Autodesk Inventor part; units mm, degrees
ref_plane "Work Plane1" through (0, 7.749, 0) normal (0, 1, 0) x (-1, 0, 0)
ref_plane "Work Plane2" through (0, 16.1, 0) normal (0, 1, 0) x (-1, 0, 0)
ref_plane "Work Plane3" through (0, 113.3, 0) normal (0, 1, 0) x (-1, 0, 0)
sketch "Sketch1" plane through (0, 0, 0) normal (0, 1, 0) x (-1, 0, 0)
  circle A0 centre (0, 0) radius 28.5
  circle A1 centre (0, 0) radius 31.877
  dimension "d0" = 57
  dimension "d1" = 63.754
extrude "Extrusion1" add sketch "Sketch1" along normal blind 114.2
ref_plane "Work Plane1" through (0, 7.749, 0) normal (0, 1, 0) x (-1, 0, 0)
sketch "Sketch3" plane through (0, 7.749, 0) normal (0, 1, 0) x (-1, 0, 0)
  circle A0 centre (0, 0) radius 31.877
  circle A1 centre (0, 0) radius 30.988
  dimension "d6" = 61.976
extrude "Extrusion2" cut sketch "Sketch3" along normal blind 200
ref_plane "Work Plane2" through (0, 16.1, 0) normal (0, 1, 0) x (-1, 0, 0)
sketch "Sketch4" plane through (0, 16.1, 0) normal (0, 1, 0) x (-1, 0, 0)
  circle A0 centre (0, 0) radius 29.5
  circle A1 centre (0, 0) radius 27.8909
  circle A2 centre (0, 0) radius 33.2417
  dimension "d10" = 59
extrude "Extrusion3" cut sketch "Sketch4" along normal blind 200 contours A2
ref_plane "Work Plane3" through (0, 113.3, 0) normal (0, 1, 0) x (-1, 0, 0)
properties part number "Vacuum Cylinder"
The listing builds one solid part. Answer for the finished solid, in the listing's coordinates (mm). A direction names the side the tool comes from. Round coordinates to 2 decimals unless told otherwise and drop trailing zeros. Order: outer loops, then holes, each group sorted by start corner. A loop starts at its lowest first (then second) coordinate and runs counter-clockwise, first axis right, second up. Notation, with made-up numbers: (29.5, 77) -> (54.5, 77) arc R22 cw to (54.5, 102) -> close; hole circle Ø6 at (35, -11.5). An arc over 180 degrees is marked (long way). Put each result on its own line as item: value.
Q1. Section B-B, the plane x = 0 is taken. Write down the section's boundary in (y, z).
Results list:
outline: (0, -31.88) -> (7.75, -31.88) -> (7.75, -30.99) -> (16.1, -30.99) -> (16.1, -29.5) -> (114.2, -29.5) -> (114.2, -28.5) -> (0, -28.5) -> close; (0, 28.5) -> (114.2, 28.5) -> (114.2, 29.5) -> (16.1, 29.5) -> (16.1, 30.99) -> (7.75, 30.99) -> (7.75, 31.88) -> (0, 31.88) -> close
Q2. Section A-A, the plane z = 0 is taken. Write down the section's boundary in (x, y).
Results list:
outline: (-31.88, 0) -> (-28.5, 0) -> (-28.5, 114.2) -> (-29.5, 114.2) -> (-29.5, 16.1) -> (-30.99, 16.1) -> (-30.99, 7.75) -> (-31.88, 7.75) -> close; (28.5, 0) -> (31.88, 0) -> (31.88, 7.75) -> (30.99, 7.75) -> (30.99, 16.1) -> (29.5, 16.1) -> (29.5, 114.2) -> (28.5, 114.2) -> close
Q3. Each of these flat-tipped pins is pushed along its axis until it touches: P1, Ø4, axis at y = 31.5, z = 18, coming from the +X side; P2, Ø4, axis at x = 18, y = 76, coming from the +Z side; P3, Ø1.5, axis at x = -3.5, y = 100.5, coming from the +Z side; P4, Ø10, axis at x = -3, z = 20, coming from the -Y side. Where does it stop, or does it pass through?
Results list:
P1: x = 24.78
P2: z = 24.78
P3: z = 29.37
P4: through
Q4. Section C-C, the plane y = 49 is taken. Write down the section's boundary in (x, z), and give its area (3 significant figures).
Results list:
outline: circle Ø59 at (0, 0); hole circle Ø57 at (0, 0)
area: 182 mm^2
Q5. Consider line 1 along Z through (x, y) = (0, 72.5); line 2 along X through (y, z) = (107, 20); line 3 along X through (y, z) = (70, 23.5). Determine where each line is inside the solid, lowest interval first.
Results list:
line 1: -29.5 to -28.5, 28.5 to 29.5
line 2: -21.69 to -20.3, 20.3 to 21.69
line 3: -17.83 to -16.12, 16.12 to 17.83
Q6. Which of the six approach directions +Z, -Z, +X, -X, +Y, -Y give full straight-line access (tool end or side, diameter ignored) to faces 1 (the flat face through (31, 7.749, 5)), 2 (the flat face through (24, 0, -16))?
Results list:
face 1: +Y
face 2: +Z, -Z, +X, -X, -Y
Q7. Determine the mould class of faces 3 (the cylindrical face through (-30.405, 3.82, -9.575)), 4 (the cylindrical face through (-26.327, 56.301, 10.916)), 5 (the flat face through (-27.4, 16.1, -11.33)) for opening direction X: pulls with the +X half, pulls with the -X half, needs draft (parallel to the pull), parting line crosses it, or undercut.
Results list:
face 3: parting line crosses it
face 4: undercut
face 5: needs draft
